Part model, mm, in its own coordinate system. A direction names the side the tool comes from. Round coordinates to 2 decimals unless told otherwise and drop trailing zeros. Order: outer loops, then holes, each group sorted by start corner. A loop starts at its lowest first (then second) coordinate and runs counter-clockwise, first axis right, second up. Notation, with made-up numbers: (33, -9.75) -> (68, -9.75) arc R15 cw to (68, 13.25) -> close; hole circle Ø11 at (62, -28). An arc over 180 degrees is marked (long way). Use CSV: the item, a comma, the result in double quotes.
```python
from build123d import *

# Parameters (mm, degrees)
BASE_FLANGE1_DEPTH     = 3
SKETCHED_BEND2_DEPTH   = 140
SKETCHED_BEND2_2_DEPTH = 140


# Read off the part's stored shape, not the designer's step: Sketched Bend2
# Sheet-metal steps are written as plain solids
with BuildPart() as part:
    # Sketch1 → Base-Flange1 (new body)
    with BuildSketch(Plane.XY):
        Polygon((0, 0), (0, 140), (47, 140), (30, 157), (30, 177), (51, 198), (215, 198), (231, 182), (231, 140), (269, 140), (269, 0), (231, 0), (231, -42), (215, -58), (51, -58), (30, -37), (30, -17), (47, 0), align=None)
    extrude(amount=-BASE_FLANGE1_DEPTH)

    # Sketched Bend2 outline → Sketched Bend2 (cut)
    with BuildSketch(Plane(origin=(0, 0, 0), x_dir=(1, 0, 0), z_dir=(0, 1, 0))):
        with BuildLine():
            Line((18.330560369, 0), (20.236135568, 1.905575199))
            ThreePointArc((20.236135568, 1.905575199), (21.448375853, 2.715568261), (22.878310766, 3))
            Line((22.878310766, 3), (0, 3))
            Line((0, 3), (0, 0))
            Line((0, 0), (18.330560369, 0))
        make_face()
    extrude(amount=SKETCHED_BEND2_DEPTH, mode=Mode.SUBTRACT)

    # Sketched Bend2 2 outline → Sketched Bend2 2 (add)
    with BuildSketch(Plane(origin=(0, 0, 0), x_dir=(1, 0, 0), z_dir=(0, 1, 0))):
        with BuildLine():
            Line((22.878310766, 0), (18.330560369, 0))
            Line((18.330560369, 0), (5.30084588, -13.029714489))
            Line((5.30084588, -13.029714489), (7.422166224, -15.151034832))
            Line((7.422166224, -15.151034832), (22.357455911, -0.215745145))
            ThreePointArc((22.357455911, -0.215745145), (22.59642615, -0.056070336), (22.878310766, 0))
        make_face()
    extrude(amount=SKETCHED_BEND2_2_DEPTH)


solid = part.part
```
(1) Pull direction Y, two halves, no side cores. Call faces 4 (the face through (26, 140, -1)), 5 (the face through (12.87, 69.02, 5.46)), 6 (the face through (223, -50, -1)), 7 (the face through (223, 190, -1)): released by +Y, released by -Y, zero draft, split by the parting line, or undercut.
Reply:
face 4,"undercut"
face 5,"zero draft"
face 6,"released by -Y"
face 7,"released by +Y"
(2) Cut at C-C, the plane z = 5.5. Give the cut face in (x, y).
Reply:
outline,"(12.83, 0) -> (17.07, 0) -> (17.07, 140) -> (12.83, 140) -> close"
(3) Which spindle directions (+Z, -Z, +X, -X, +Y, -Y) get a long thin tool onto all of the face, cutting with end or side? Do faces 1 (the face through (148, 72, 0)), 2 (the face through (39, 148, -1)), 3 (the face through (148, 72, -3)). Say none if no direction does.
Reply:
face 1,"+Z, +X, +Y, -Y"
face 2,"+Z, -Z, -X"
face 3,"-Z, +X, -X, +Y, -Y"
(4) Cut at B-B, the plane x = 251. Give the cut face in (y, z).
Reply:
outline,"(0, -3) -> (140, -3) -> (140, 0) -> (0, 0) -> close"
(5) Cut at A-A, the plane y = 37. Give the cut face in (x, z).
Reply:
outline,"(5.3, 13.03) -> (20.24, -1.91) arc R3.74 ccw to (22.88, -3) -> (269, -3) -> (269, 0) -> (22.88, 0) arc R0.74 cw to (22.36, 0.22) -> (7.42, 15.15) -> close"
(6) Drop flat-ended pins along their axis: P1, Ø1.5, axis at y = 163, z = -1, coming from the +X side; P2, Ø0.9, axis at y = -25, z = -1.5, coming from the -X side; P3, Ø8, axis at y = 73, z = 13, coming from the -X side; P4, Ø3, axis at x = 36.5, z = 2, coming from the -Y side. Give the stop position or say it passes through.
Reply:
P1,"x = 231"
P2,"x = 30"
P3,"x = 5.3"
P4,"through"
(7) Probe probe 1 along Z at (x, y) = (158, 176); probe 2 along X at (y, z) = (101, 3.75); probe 3 along X at (y, z) = (99, 12.75). List the from-to ranges inside material, lowest first. Write a range as [from, to].
Reply:
probe 1,"[-3, 0]"
probe 2,"[14.58, 18.82]"
probe 3,"[5.58, 9.82]"
